Autodesk Inventor part; units mm, degrees
ref_plane "YZ Plane" through (0, 0, 0) normal (1, 0, 0) x (0, 1, 0)
ref_plane "XZ Plane" through (0, 0, 0) normal (0, 1, 0) x (-1, 0, 0)
ref_plane "XY Plane" through (0, 0, 0) normal (0, 0, 1) x (1, 0, 0)
sketch "Boceto1" plane through (0, 0, 0) normal (0, 0, 1) x (1, 0, 0)
  circle A0 centre (0, 0) radius 2.5
  dimension "d1" = 5
extrude "Extrusión1" add sketch "Boceto1" along normal blind 513
sketch "Boceto2" plane through (0, 0, 0) normal (1, 0, 0) x (0, 1, 0)
  line L0 (0, 0) -> (0, 8.92)
  line L1 (0, 8.92) -> (-2.5, 8.92)
  line L2 (-2.5, 0) -> (-2.5, 513)
  line L3 (-2.5, 0) -> (-2.5, 513)
  line L4 (-2.5, 8.42) -> (-2, 8.42)
  line L5 (-2, 8.42) -> (-2, 9.42)
  line L6 (-2, 9.42) -> (-2.5, 9.42)
  line L7 (-2.5, 9.42) -> (-2.5, 8.42)
  dimension "d4" = 8.92
revolve "Revolución1" cut sketch "Boceto2" angle 360 about axis through (0, 0, 0) along (0, 0, 1)
sketch "Boceto3" plane through (0, 0, 0) normal (1, 0, 0) x (0, 1, 0)
  line L0 (2.5, 513) -> (-2.5, 513)
  line L1 (0, 513) -> (0, 503.5)
  line L2 (0, 503.5) -> (-2.5, 503.5)
  line L3 (-2.5, 9.42) -> (-2.5, 513)
  line L4 (-2.5, 503.5) -> (-2, 503.5)
  line L5 (-2, 503.5) -> (-2, 503)
  line L6 (-2, 503) -> (-2.5, 503)
  line L7 (-2.5, 503) -> (-2.5, 503.5)
  line L8 (-2.5, 503.5) -> (-2, 503.5)
  line L9 (-2, 503.5) -> (-2, 504)
  line L10 (-2, 504) -> (-2.5, 504)
  line L11 (-2.5, 504) -> (-2.5, 503.5)
  point P0 (0, 0)
  dimension "d8" = 9.5
  dimension "d9" = 0.5
  dimension "d10" = 0.5
  dimension "d11" = 0.5
  dimension "d12" = 0.5
revolve "Revolución2" cut sketch "Boceto3" angle 360 about axis through (0, 0, 513) along (0, 0, -1) contours L10 L9 L2 L3 | L5 L6 L3 L2
properties part number "union"
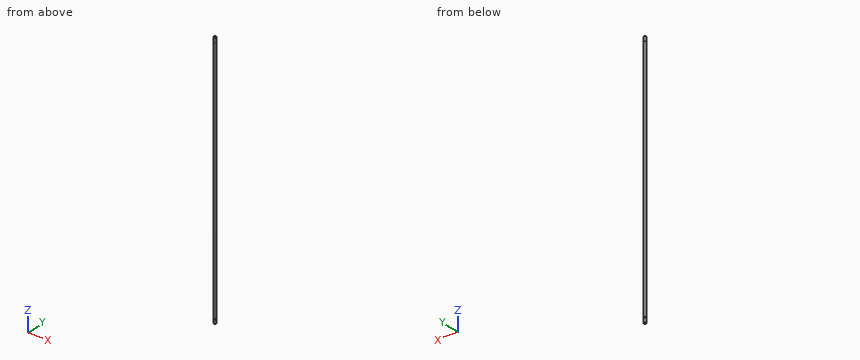
Work out the finished part from the listing and answer in its coordinate system (mm). Give positions to 0.01 mm unless a question says otherwise; leave off trailing zeros. Loops run counter-clockwise (first coordinate to the right, second up) from the corner with the lowest first, then second, coordinate; pieces in that order, holes last. Notation, with made-up numbers: (88, 32.5) - (145, 32.5) arc R16 ccw to (145, 37.5) - close; hole circle Ø5 at (47, -25). An arc over 180 degrees is marked (long way). Answer in a Markdown table with one row per item. Add a question column.
Q1. The part is cut by section B-B (x = 0.75). Determine the outline of the cut face in (y, z), and give its area (3 significant figures).
Q2. The part is cut by section C-C (z = 104.5). Determine the outline of the cut face in (x, y), and give its area (3 significant figures).
Q3. This flat-tipped pin is pushed along its axis until it touches: P1, Ø1, axis at y = 1.5, z = 373.5, coming from the +X side. Where does it stop, or does it pass through?
Q4. The part is cut by section A-A (y = -1.15). Determine the outline of the cut face in (x, z), and give its area (3 significant figures).
Q5. Consider line 1 along Y through (x, z) = (1.45, 94); line 2 along Y through (x, z) = (-1.6, 344); line 3 along X through (y, z) = (-1.5, 218.5). Determine where each line is inside the solid, lowest interval first.
Solution:
| question | item | result |
|---|---|---|
| 1 | outline | (-2.38, 0) - (2.38, 0) - (2.38, 8.42) - (1.85, 8.42) - (1.85, 9.42) - (2.38, 9.42) - (2.38, 503) - (1.85, 503) - (1.85, 504) - (2.38, 504) - (2.38, 513) - (-2.38, 513) - (-2.38, 504) - (-1.85, 504) - (-1.85, 503) - (-2.38, 503) - (-2.38, 9.42) - (-1.85, 9.42) - (-1.85, 8.42) - (-2.38, 8.42) - close |
| 1 | area | 2,440 mm² |
| 2 | outline | circle Ø5 at (0, 0) |
| 2 | area | 19.6 mm² |
| 3 | P1 | stops at x = 2.29 |
| 4 | outline | (-2.22, 0) - (2.22, 0) - (2.22, 8.42) - (1.64, 8.42) - (1.64, 9.42) - (2.22, 9.42) - (2.22, 503) - (1.64, 503) - (1.64, 504) - (2.22, 504) - (2.22, 513) - (-2.22, 513) - (-2.22, 504) - (-1.64, 504) - (-1.64, 503) - (-2.22, 503) - (-2.22, 9.42) - (-1.64, 9.42) - (-1.64, 8.42) - (-2.22, 8.42) - close |
| 4 | area | 2,280 mm² |
| 5 | line 1 | y = -2.04 to 2.04 |
| 5 | line 2 | y = -1.92 to 1.92 |
| 5 | line 3 | x = -2 to 2 |
